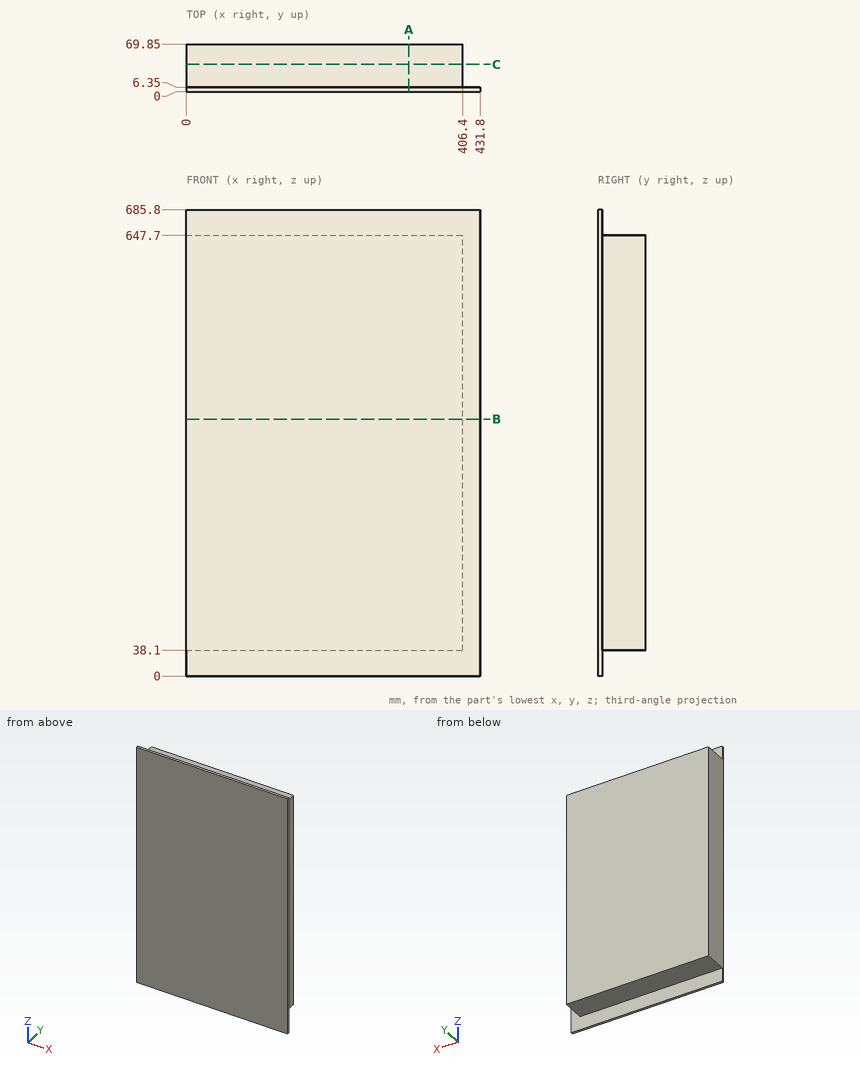
Can you work these out from the drawing? Everything is in mm from the part's minimum corner. Coordinates: 2 decimals unless noted, no trailing zeros. Order: outer loops, then holes, each group sorted by start corner. A loop starts at its lowest first (then second) coordinate and runs counter-clockwise, first axis right, second up. Notation, with made-up numbers: M 73,-3.75 L 108,-3.75 A18 cw 108,1.25 Z; hole C 26,27 d7. An arc over 180 degrees is marked long. Answer as CSV lines item,"result". Start each with the question number.
1. I need wall thicknesses on line 1 (X direction, y = 10, z = 90); line 2 (Z direction, x = 307, y = 62.5). Which ranges of each line are inside material? Lowest first, please. Write a range as [from, to].
2. I want a section at C-C, the plane y = 40. Write out the boundary of the cut face in (x, z).
3. I want a section at A-A, the plane x = 327. Write out the boundary of the cut face in (y, z).
4. I want a section at B-B, the plane z = 377.5. Write out the boundary of the cut face in (x, y), and give its area (3 significant figures).
5. For pin 1 (2 mm diameter, centred on x = 173, y = 53, fed in from -Z); pin 2 (19 mm diameter, centred on y = 29, z = 479, fed in from +X); pin 3 (12 mm diameter, centred on x = 282.5, y = 60, fed in from +Z), each with a flat end and sliding along its axis, tell me the tip position at first contact or that it passes through.
Recorded:
1,line 1,"x = [0, 406.4]"
1,line 2,"z = [38.1, 647.7]"
2,outline,"M 0,38.1 L 406.4,38.1 L 406.4,647.7 L 0,647.7 Z"
3,outline,"M 0,0 L 6.35,0 L 6.35,38.1 L 69.85,38.1 L 69.85,647.7 L 6.35,647.7 L 6.35,685.8 L 0,685.8 Z"
4,outline,"M 0,0 L 431.8,0 L 431.8,6.35 L 406.4,6.35 L 406.4,69.85 L 0,69.85 Z"
4,area,"28,500 mm2"
5,pin 1,"stops at z = 38.1"
5,pin 2,"stops at x = 406.4"
5,pin 3,"stops at z = 647.7"
